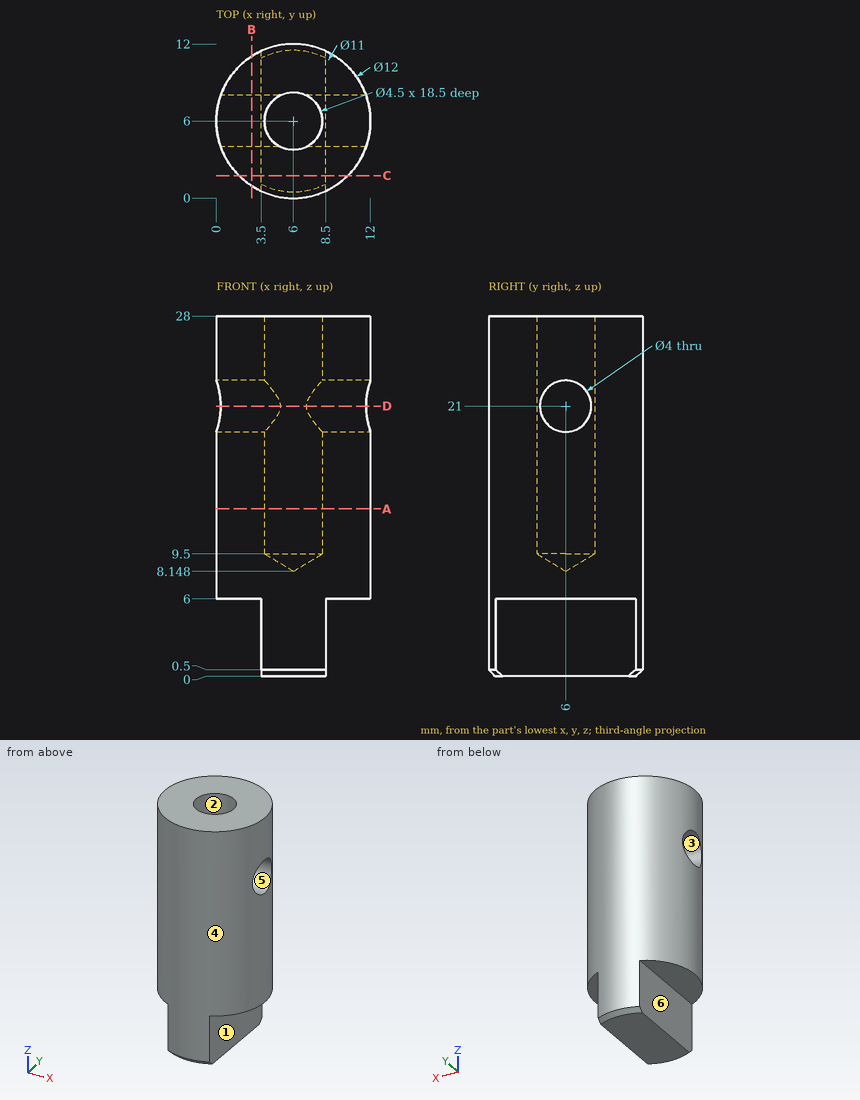
Geometry: see drawing. Coordinates: mm, zero at the bounding-box minimum. A direction names the side the tool comes from. Give positions to 0.01 mm unless a question says otherwise; leave off trailing zeros. Loops run counter-clockwise (first coordinate to the right, second up) from the corner with the lowest first, then second, coordinate; pieces in that order, holes last. Notation, with made-up numbers: (35.25, -37) -> (83.25, -37) arc R29 ccw to (83.25, -4) -> close; hole circle Ø8 at (86, 30). An arc over 180 degrees is marked (long way). Use one line per item in the form item = value.
Item 1: Pin query (flat end, axial travel): P1, Ø1.5, axis at y = 9, z = 11.5, coming from the -X side; P2, Ø5, axis at x = 2, z = 21, coming from the +Y side; P3, Ø3.5, axis at y = 6, z = 21, coming from the -X side; P4, Ø5, axis at y = 3.5, z = 3, coming from the -X side. Return the tip coordinate at first contact, or that it passes through.
A:
P1 = 0.44
P2 = 11.81
P3 = through
P4 = 3.5
Item 2: Section query C-C on y = 1.75. Output: boundary loops of the cut face in (x, z), and give its area (3 significant figures).
A:
outline = (1.76, 6) -> (3.5, 6) -> (3.5, 0) -> (8.5, 0) -> (8.5, 6) -> (10.24, 6) -> (10.24, 28) -> (1.76, 28) -> close
area = 216 mm^2
Item 3: Draft query along Y for the marked faces 1, 2, 3 and 4. Return one class per face: pulls with the +Y half, pulls with the -Y half, needs draft (parallel to the pull), parting line crosses it, or undercut.
A:
face_1 = needs draft
face_2 = undercut
face_3 = undercut
face_4 = parting line crosses it
Item 4: Section query A-A on z = 13. Output: boundary loops of the cut face in (x, y).
A:
outline = circle Ø12 at (6, 6); hole circle Ø4.5 at (6, 6)
Item 5: Section query B-B on x = 2.75. Output: boundary loops of the cut face in (y, z), and give its area (3 significant figures).
A:
outline = (0.96, 6) -> (11.04, 6) -> (11.04, 28) -> (0.96, 28) -> close; hole circle Ø4 at (6, 21)
area = 209 mm^2
Item 6: Access query for the marked faces 5 and 6. Directions: +Z, -Z, +X, -X, +Y, -Y. A direction counts if a zero-diameter tool reaches every point of the face in a straight line with its end or side. Return the directions, or none.
A:
face_5 = +X, -X
face_6 = -Z, -X, +Y, -Y
Item 7: Section query D-D on z = 21. Output: boundary loops of the cut face in (x, y).
A:
outline = (0.34, 4) arc R6 ccw to (11.66, 4) -> (7.03, 4) arc R2.25 cw to (4.97, 4) -> close; (0.34, 8) -> (4.97, 8) arc R2.25 cw to (7.03, 8) -> (11.66, 8) arc R6 ccw to start
Item 8: Line query: probe 1 along Y at (x, z) = (6, 17.75); probe 2 along Y at (x, z) = (8.4, 21); probe 3 along X at (y, z) = (6.75, 3.75). Output: solid intervals per line, ascending.
A:
probe_1 = 0 to 3.75, 8.25 to 12
probe_2 = 0.5 to 4, 8 to 11.5
probe_3 = 3.5 to 8.5
